Answer from the drawing. Dimensions are ordinates in mm from the lowest x, y and z of the part. Coordinates: 2 decimals unless noted, no trailing zeros. Loops run counter-clockwise (first coordinate to the right, second up) from the corner with the lowest first, then second, coordinate; pieces in that order, holes last.
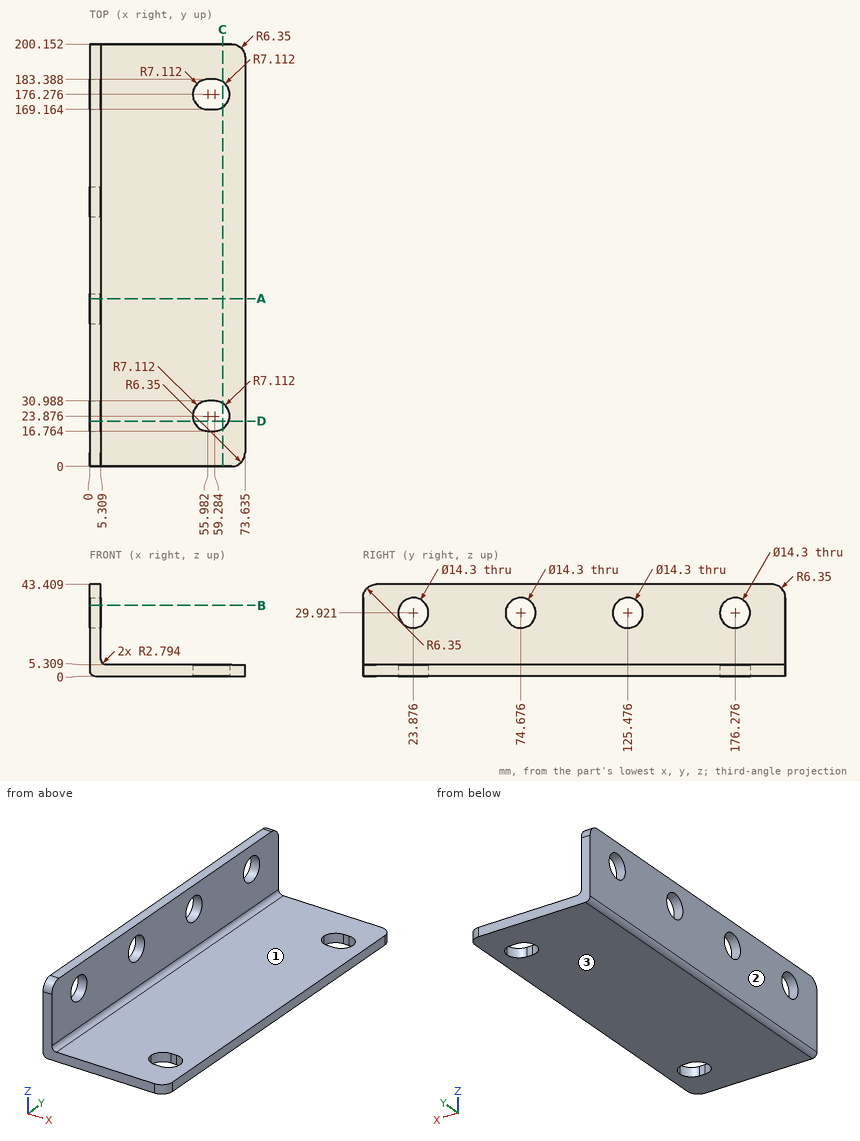
Item 1: A cutting plane is placed at D-D on y = 21.5. Determine the outline of the cut face in (x, z) (1 decimal), then the cut area to 3 significant figures.
Numbers:
outline: (0, 2.8) arc R2.8 ccw to (2.8, 0) - (49.3, 0) - (49.3, 5.3) - (8.1, 5.3) arc R2.8 cw to (5.3, 8.1) - (5.3, 23.2) - (0, 23.2) - close; (0, 36.7) - (5.3, 36.7) - (5.3, 43.4) - (0, 43.4) - close; (66, 0) - (73.6, 0) - (73.6, 5.3) - (66, 5.3) - close
area: 433 mm2
Item 2: A cutting plane is placed at A-A on y = 79.5. Determine the outline of the cut face in (x, z) (1 decimal).
Numbers:
outline: (0, 2.8) arc R2.8 ccw to (2.8, 0) - (73.6, 0) - (73.6, 5.3) - (8.1, 5.3) arc R2.8 cw to (5.3, 8.1) - (5.3, 24.6) - (0, 24.6) - close; (0, 35.2) - (5.3, 35.2) - (5.3, 43.4) - (0, 43.4) - close
Item 3: A cutting plane is placed at C-C on x = 63. Determine the outline of the cut face in (y, z).
Numbers:
outline: (0, 0) - (17.81, 0) - (17.81, 5.31) - (0, 5.31) - close; (29.94, 0) - (170.21, 0) - (170.21, 5.31) - (29.94, 5.31) - close; (182.34, 0) - (200.15, 0) - (200.15, 5.31) - (182.34, 5.31) - close
Item 4: A cutting plane is placed at B-B on z = 33.5. Determine the outline of the cut face in (x, y).
Numbers:
outline: (0, 0) - (5.31, 0) - (5.31, 17.69) - (0, 17.69) - close; (0, 30.07) - (5.31, 30.07) - (5.31, 68.49) - (0, 68.49) - close; (0, 80.87) - (5.31, 80.87) - (5.31, 119.29) - (0, 119.29) - close; (0, 131.67) - (5.31, 131.67) - (5.31, 170.09) - (0, 170.09) - close; (0, 182.47) - (5.31, 182.47) - (5.31, 200.15) - (0, 200.15) - close
Item 5: Given pin 1 (6 mm diameter, centred on x = 25, y = 167.5, fed in from +Z); pin 2 (8.5 mm diameter, centred on y = 74.68, z = 29.92, fed in from -X); pin 3 (16.5 mm diameter, centred on y = 125.48, z = 29.92, fed in from +X), each flat-ended and moving along its own axis, determine where each tip first touches the part or whether it passes through.
Numbers:
pin 1: stops at z = 5.31
pin 2: passes through
pin 3: stops at x = 5.31
Item 6: Find the intervals of material crossed by line 1 along X through (y, z) = (153, 26); line 2 along Z through (x, y) = (7, 142) (1 decimal), in increasing order.
Numbers:
line 1: x = 0 to 5.31
line 2: z = 0 to 5.5
Item 7: Determine the mould class of the marked faces 1, 2 and 3 for opening direction Z: released by +Z, released by -Z, zero draft, split by the parting line, or undercut.
Numbers:
face 1: released by +Z
face 2: zero draft
face 3: released by -Z
